Source: CAD feature listing. Evaluate the final solid. Frame: model axes, mm. Face numbers are marked on the shaded views. A direction names the side the tool comes from. Coordinates: 2 decimals unless noted, no trailing zeros. Loops run counter-clockwise (first coordinate to the right, second up) from the corner with the lowest first, then second, coordinate; pieces in that order, holes last. Notation, with made-up numbers: (-39, 55) - (-19, 55) arc R21 cw to (-19, 77) - close; hole circle Ø9 at (-9, 86.25). An arc over 180 degrees is marked (long way). Use one line per item in the form item = value. Start each with the question number.
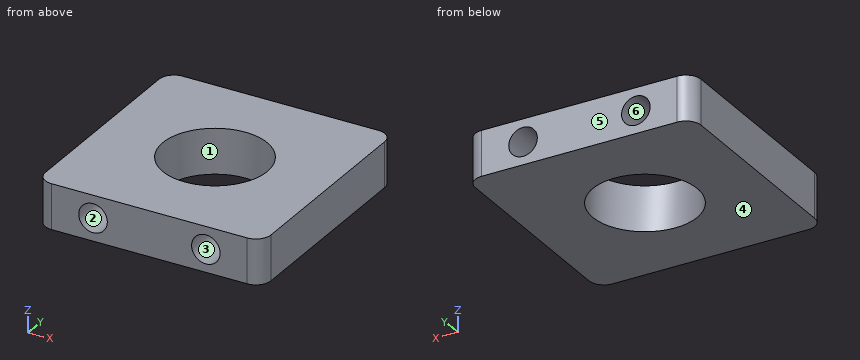
from build123d import *

# Parameters (mm, degrees)
SKETCH1_W           = 38.1
SKETCH1_H           = 38.1
SKETCH1_R           = 8.8265
BOSS_EXTRUDE1_DEPTH = 7.62
FILLET1_R           = 2.54
SKETCH2_R           = 2.413
CUT_EXTRUDE1_DEPTH  = 7.62
SKETCH3_R           = 2.413
CUT_EXTRUDE2_DEPTH  = 7.62


with BuildPart() as part:
    # Sketch1 → Boss-Extrude1 (new body)
    with BuildSketch(Plane.XY):
        Rectangle(SKETCH1_W, SKETCH1_H)
        Circle(SKETCH1_R, mode=Mode.SUBTRACT)
    extrude(amount=BOSS_EXTRUDE1_DEPTH)

    # Fillet1
    fillet1_edges = [part.edges().sort_by_distance(p)[0] for p in [
        (-19.05, 19.05, 3.81),
        (19.05, 19.05, 3.81),
        (19.05, -19.05, 3.81),
        (-19.05, -19.05, 3.81),
    ]]
    fillet(fillet1_edges, radius=FILLET1_R)

    # Sketch2 → Cut-Extrude1 (cut)
    with BuildSketch(Plane.XZ.offset(19.05)):
        with Locations((9.525, 3.81)):
            Circle(SKETCH2_R)
        with Locations((-9.525, 3.81)):
            Circle(SKETCH2_R)
    extrude(amount=-CUT_EXTRUDE1_DEPTH, mode=Mode.SUBTRACT)

    # Sketch3 → Cut-Extrude2 (cut)
    with BuildSketch(Plane(origin=(0, 19.05, 0), x_dir=(1, 0, 0), z_dir=(0, 1, 0))):
        with Locations((-9.525, -3.81)):
            Circle(SKETCH3_R)
        with Locations((9.525, -3.81)):
            Circle(SKETCH3_R)
    extrude(amount=-CUT_EXTRUDE2_DEPTH, mode=Mode.SUBTRACT)


solid = part.part
(1) Cut plane A-A, the plane x = 0. Output: boundary loops of the cut face in (y, z).
(2) Contact query for flat-ended pins moving along their axis: pin 1 (2.5 mm diameter, centred on x = 10, z = 4, fed in from -Y); pin 2 (4 mm diameter, centred on x = -9.525, z = 3.81, fed in from +Y); pin 3 (3 mm diameter, centred on x = -3.5, y = -10.5, fed in from -Z); pin 4 (14 mm diameter, centred on x = 0, y = 0, fed in from -Z). Output: stop coordinate, or through.
(3) Material intervals for line 1 (X direction, y = 15.25, z = 3.81); line 2 (Y direction, x = 0, z = 2); line 3 (Y direction, x = -1.5, z = 1), sorted ascending.
(4) Cut plane C-C, the plane z = 3.81. Output: boundary loops of the cut face in (x, y).
(5) Cut plane D-D, the plane y = 3. Output: boundary loops of the cut face in (x, z).
(6) Cut plane B-B, the plane y = 15. Output: boundary loops of the cut face in (x, z) (3 decimals).
(7) Access query for the marked faces 5 and 6. Directions: +Z, -Z, +X, -X, +Y, -Y. A direction counts if a zero-diameter tool reaches every point of the face in a straight line with its end or side. Return the directions, or none.
(8) Mould query, pull axis Z, two halves, no side actions, for the marked faces 1, 2, 3 and 4. Classes: +Z half, -Z half, draft (parallel to the pull), parting line (faces both ways), or undercut.
Recorded:
q1.outline = (-19.05, 0) - (-8.83, 0) - (-8.83, 7.62) - (-19.05, 7.62) - close; (8.83, 0) - (19.05, 0) - (19.05, 7.62) - (8.83, 7.62) - close
q2.pin_1 = -11.43
q2.pin_2 = 11.43
q2.pin_3 = 0
q2.pin_4 = through
q3.line_1 = -19.05 to -11.94, -7.11 to 7.11, 11.94 to 19.05
q3.line_2 = -19.05 to -8.83, 8.83 to 19.05
q3.line_3 = -19.05 to -8.7, 8.7 to 19.05
q4.outline = (-19.05, -16.51) arc R2.54 ccw to (-16.51, -19.05) - (-11.94, -19.05) - (-11.94, -11.43) - (-7.11, -11.43) - (-7.11, -19.05) - (7.11, -19.05) - (7.11, -11.43) - (11.94, -11.43) - (11.94, -19.05) - (16.51, -19.05) arc R2.54 ccw to (19.05, -16.51) - (19.05, 16.51) arc R2.54 ccw to (16.51, 19.05) - (11.94, 19.05) - (11.94, 11.43) - (7.11, 11.43) - (7.11, 19.05) - (-7.11, 19.05) - (-7.11, 11.43) - (-11.94, 11.43) - (-11.94, 19.05) - (-16.51, 19.05) arc R2.54 ccw to (-19.05, 16.51) - close; hole circle Ø17.65 at (0, 0)
q5.outline = (-19.05, 0) - (-8.3, 0) - (-8.3, 7.62) - (-19.05, 7.62) - close; (8.3, 0) - (19.05, 0) - (19.05, 7.62) - (8.3, 7.62) - close
q6.outline = (-19.05, 0) - (19.05, 0) - (19.05, 7.62) - (-19.05, 7.62) - close; hole circle Ø4.826 at (-9.525, 3.81); hole circle Ø4.826 at (9.525, 3.81)
q7.face_5 = +Z, -Z, +X, -X, +Y
q7.face_6 = +Y
q8.face_1 = draft
q8.face_2 = undercut
q8.face_3 = undercut
q8.face_4 = -Z half
